Geometry check sheet. Reference: the model listing, model coordinates, mm. Face numbers are marked on the shaded views. Coordinates: 2 decimals unless noted, no trailing zeros. Loops run counter-clockwise (first coordinate to the right, second up) from the corner with the lowest first, then second, coordinate; pieces in that order, holes last.
from build123d import *

# Parameters (mm, degrees)
SKETCH1_W           = 85.852
SKETCH1_H           = 101.6
BOSS_EXTRUDE1_DEPTH = 12.7
SHELL1_T            = -10.16
SKETCH3_R           = 2.54
SKETCH3_R_2         = 0.762
BOSS_EXTRUDE7_DEPTH = 3.81
FILLET1_R           = 5.08
CUT_EXTRUDE4_START  = -7.62
CUT_EXTRUDE4_DEPTH  = 7.62
SKETCH10_R          = 3.81
SKETCH10_R_2        = 1.905
BOSS_EXTRUDE6_DEPTH = 27.94
CUT_EXTRUDE5_DEPTH  = 83.058
SKETCH13_R          = 1.905
SKETCH13_R_2        = 0.762
CUT_EXTRUDE6_DEPTH  = 9.906


with BuildPart() as part:
    # Sketch1 → Boss-Extrude1 (new body)
    with BuildSketch(Plane.XY):
        Rectangle(SKETCH1_W, SKETCH1_H)
    extrude(amount=BOSS_EXTRUDE1_DEPTH)

    # Shell1
    shell1_openings = [part.faces().sort_by_distance(p)[0] for p in [
        (0, 0, 12.7),
    ]]
    offset(amount=SHELL1_T, openings=shell1_openings, kind=Kind.INTERSECTION)

    # Sketch3 → Boss-Extrude7 (add)
    # profile 1 of 4: a face of its own
    with BuildSketch(Plane.XY.offset(10.16)):
        with Locations(Location((-19.139245454, 33.606248823, 0), (0, 0, 180))):
            Circle(SKETCH3_R)
        with Locations(Location((-19.139245454, 33.606248823, 0), (0, 0, 180))):
            Circle(SKETCH3_R_2, mode=Mode.SUBTRACT)
    # profile 2 of 4: a face of its own
    with BuildSketch(Plane.XY.offset(10.16)):
        with Locations(Location((29.860754546, 33.606248823, 0), (0, 0, 180))):
            Circle(SKETCH3_R)
        with Locations(Location((29.860754546, 33.606248823, 0), (0, 0, 180))):
            Circle(SKETCH3_R_2, mode=Mode.SUBTRACT)
    # profile 3 of 4: a face of its own
    with BuildSketch(Plane.XY.offset(10.16)):
        with Locations(Location((29.860754546, -24.393751177, 0), (0, 0, 180))):
            Circle(SKETCH3_R)
        with Locations(Location((29.860754546, -24.393751177, 0), (0, 0, 180))):
            Circle(SKETCH3_R_2, mode=Mode.SUBTRACT)
    # profile 4 of 4: a face of its own
    with BuildSketch(Plane.XY.offset(10.16)):
        with Locations(Location((-19.139245454, -24.393751177, 0), (0, 0, 180))):
            Circle(SKETCH3_R)
        with Locations(Location((-19.139245454, -24.393751177, 0), (0, 0, 180))):
            Circle(SKETCH3_R_2, mode=Mode.SUBTRACT)
    extrude(amount=BOSS_EXTRUDE7_DEPTH)

    # Fillet1
    fillet1_edges = [part.edges().sort_by_distance(p)[0] for p in [
        (-42.926, 50.8, 6.35),
        (42.926, 50.8, 6.35),
        (42.926, -50.8, 6.35),
        (-42.926, -50.8, 6.35),
    ]]
    fillet(fillet1_edges, radius=FILLET1_R)

    # Sketch7 → Cut-Extrude4 (cut)
    with BuildSketch(Plane(origin=(0, 0, 0), x_dir=(-1, 0, 0), z_dir=(0, 0, -1)).offset(CUT_EXTRUDE4_START)):
        with BuildLine():
            Line((-37.846, -50.8), (37.846, -50.8))
            ThreePointArc((37.846, -50.8), (41.438102448, -49.312102448), (42.926, -45.72))
            Line((42.926, -45.72), (42.926, 45.72))
            ThreePointArc((42.926, 45.72), (41.438102448, 49.312102448), (37.846, 50.8))
            Line((37.846, 50.8), (-37.846, 50.8))
            ThreePointArc((-37.846, 50.8), (-41.438102448, 49.312102448), (-42.926, 45.72))
            Line((-42.926, 45.72), (-42.926, -45.72))
            ThreePointArc((-42.926, -45.72), (-41.438102448, -49.312102448), (-37.846, -50.8))
        make_face()
    extrude(amount=CUT_EXTRUDE4_DEPTH, mode=Mode.SUBTRACT)

    # Sketch10 → Boss-Extrude6 (add)
    # profile 1 of 4: a face of its own
    with BuildSketch(Plane.XY.offset(12.7)):
        with Locations((-38.1, 44.45)):
            Circle(SKETCH10_R)
        with Locations((-38.1, 44.45)):
            Circle(SKETCH10_R_2, mode=Mode.SUBTRACT)
    # profile 2 of 4: a face of its own
    with BuildSketch(Plane.XY.offset(12.7)):
        with Locations((38.1, 44.45)):
            Circle(SKETCH10_R)
        with Locations((38.1, 44.45)):
            Circle(SKETCH10_R_2, mode=Mode.SUBTRACT)
    # profile 3 of 4: a face of its own
    with BuildSketch(Plane.XY.offset(12.7)):
        with Locations((38.1, -44.45)):
            Circle(SKETCH10_R)
        with Locations((38.1, -44.45)):
            Circle(SKETCH10_R_2, mode=Mode.SUBTRACT)
    # profile 4 of 4: a face of its own
    with BuildSketch(Plane.XY.offset(12.7)):
        with Locations((-38.1, -44.45)):
            Circle(SKETCH10_R)
        with Locations((-38.1, -44.45)):
            Circle(SKETCH10_R_2, mode=Mode.SUBTRACT)
    extrude(amount=BOSS_EXTRUDE6_DEPTH)

    # Sketch11 → Cut-Extrude5 (cut)
    with BuildSketch(Plane.XY):
        Polygon((-38.054358592, -21.497558928), (38.145641408, -21.497558928), (38.145641408, 30.251057274), (-22.70646811, 30.251057274), (-22.70646811, 35.689101497), (-38.054358592, 35.689101497), align=None)
    extrude(amount=CUT_EXTRUDE5_DEPTH, mode=Mode.SUBTRACT)

    # Sketch13 → Cut-Extrude6 (cut)
    with BuildSketch(Plane.XY.offset(12.7)):
        with BuildLine():
            Line((-27.477284385, 42.802269742), (-27.477284385, 44.707269742))
            Line((-27.477284385, 44.707269742), (-25.572284385, 44.707269742))
            ThreePointArc((-25.572284385, 44.707269742), (-28.824322804, 46.05430816), (-27.477284385, 42.802269742))
        make_face()
        with Locations((26.520719639, 44.707269742)):
            Circle(SKETCH13_R)
        with Locations((-27.477284385, -46.187542617)):
            Circle(SKETCH13_R)
        with Locations((26.520719639, -46.187542617)):
            Circle(SKETCH13_R)
        with Locations((10.5, 48.630171944)):
            Circle(SKETCH13_R_2)
        with Locations((-10.5, 48.630171944)):
            Circle(SKETCH13_R_2)
    extrude(amount=-CUT_EXTRUDE6_DEPTH, mode=Mode.SUBTRACT)


solid = part.part
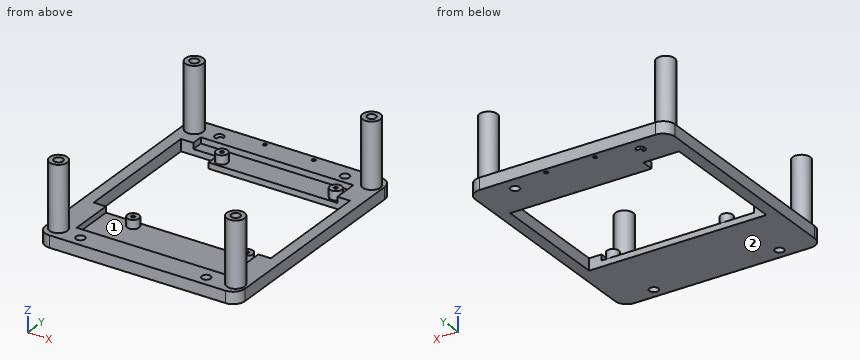
1) Section check B-B on x = 18.5. Record the cut outline in (y, z).
Data:
outline: (-50.8, 7.62) - (-21.5, 7.62) - (-21.5, 10.16) - (-40.64, 10.16) - (-40.64, 12.7) - (-50.8, 12.7) - close; (30.25, 7.62) - (50.8, 7.62) - (50.8, 12.7) - (40.64, 12.7) - (40.64, 10.16) - (30.25, 10.16) - close
2) Section check D-D on y = 38.5. Record the cut outline in (x, z).
Data:
outline: (-42.93, 7.62) - (42.93, 7.62) - (42.93, 12.7) - (32.77, 12.7) - (32.77, 10.16) - (-32.77, 10.16) - (-32.77, 12.7) - (-42.93, 12.7) - close
3) Mould release check, pull along X, two halves, no side actions. Record for the marked faces 1 and 2: +X half, -X half, draft (parallel to the pull), parting line (faces both ways), or undercut.
Data:
face 1: undercut
face 2: draft
4) Material ranges on probe 1 along X at (y, z) = (44.5, 26); probe 2 along X at (y, z) = (-14, 11); probe 3 along Y at (x, z) = (26.5, 9), recorded low to high.
Data:
probe 1: x = -41.91 to -40, -36.2 to -34.29, 34.29 to 36.2, 40 to 41.91
probe 2: x = -42.93 to -38.05, 38.15 to 42.93
probe 3: y = -50.8 to -48.09, -44.28 to -21.5, 30.25 to 42.8, 46.61 to 50.8
5) Section check C-C on y = -9. Record the cut outline in (x, z).
Data:
outline: (-42.93, 7.62) - (-38.05, 7.62) - (-38.05, 12.7) - (-42.93, 12.7) - close; (38.15, 7.62) - (42.93, 7.62) - (42.93, 12.7) - (38.15, 12.7) - close
6) Section check A-A on z = 34. Record the cut outline in (x, y) (3 decimals).
Data:
outline: circle Ø7.62 at (-38.1, -44.45); circle Ø7.62 at (-38.1, 44.45); circle Ø7.62 at (38.1, -44.45); circle Ø7.62 at (38.1, 44.45); hole circle Ø3.81 at (-38.1, -44.45); hole circle Ø3.81 at (-38.1, 44.45); hole circle Ø3.81 at (38.1, -44.45); hole circle Ø3.81 at (38.1, 44.45)
7) Depth check by flat-ended pin: pin 1 (5 mm diameter, centred on x = -33.5, z = 23, fed in from -Y); pin 2 (1.1 mm diameter, centred on x = -38.5, y = -43.5, fed in from +Z). Enter the tip coordinate at first touch or a pass-through.
Data:
pin 1: stops at y = -47.63
pin 2: stops at z = 12.7
